Can you work these out from the model? Positions are in its coordinate system, mm. A direction names the side the tool comes from. Round coordinates to 2 decimals unless told otherwise and drop trailing zeros. Loops run counter-clockwise (first coordinate to the right, second up) from the corner with the lowest first, then second, coordinate; pieces in that order, holes last.
```python
from build123d import *

# Parameters (mm, degrees)
BASE_EXTRUDE_DEPTH = 10


with BuildPart() as part:
    # Sketch1 → Base-Extrude (new body)
    with BuildSketch(Plane.XY):
        with BuildLine():
            Line((89.567268983, -20.929801144), (19.452075124, 29.096679766))
            ThreePointArc((19.452075124, 29.096679766), (-16.495110953, 30.869261648), (-35, 0))
            ThreePointArc((-35, 0), (-43.227486122, -3.818813079), (-40.833333333, 4.930066486))
            Line((-40.833333333, 4.930066486), (-41.666666667, 9.860132972))
            ThreePointArc((-41.666666667, 9.860132972), (-46.454972244, -7.637626158), (-30, 0))
            ThreePointArc((-30, 0), (-14.170913912, 26.442110334), (16.612346594, 24.980591279))
            Line((16.612346594, 24.980591279), (86.66322331, -25))
            Line((86.66322331, -25), (89.567268983, -20.929801144))
        make_face()
    extrude(amount=BASE_EXTRUDE_DEPTH)


solid = part.part
```
(1) We'd pull the mould along Y, two halves only. Please class faces 1 (the flat face through (88.095, -22.993, 4.93)), 2 (the flat face through (25, 21, 10)), 3 (the cylindrical face through (-43, -4, 5)), 4 (the cylindrical face through (-16.026, 31.115, 4.93)): released by +Y, released by -Y, zero draft, split by the parting line, or undercut.
(2) Which directions (+Z, -Z, +X, -X, +Y, -Y) give clear straight access to the entire face, cutting with the end or side of a thin tool? Please do faces 5 (the flat face through (-41.244, 7.361, 4.93)), 6 (the cylindrical face through (-46.69, -7.43, 4.93)), 7 (the flat face through (51.15, 0.34, 4.93)).
(3) For pin 1 (12 mm diameter, centred on x = 21.5, y = 28.5, fed in from +Z); pin 2 (4 mm diameter, centred on x = 47, z = 5.5, fed in from -Y); pin 3 (4 mm diameter, centred on y = 5.5, z = 5.5, fed in from -X); pin 4 (3 mm diameter, centred on x = 59.5, z = 1.5, fed in from -Y), each with a flat end and sliding along its axis, tell me the tip position at first contact or that it passes through.
(4) If I drill on line 1 (Y direction, x = -40, z = 4.25); line 2 (X direction, y = 22, z = 6.75); line 3 (X direction, y = 16, z = 2.5), over which ranges is the centre line in solid material (lowest first)?
(5) Suppose I cut it at A-A (z = 5.5). Write out the boundary of the cut face in (x, y).
(6) Suppose I cut it at B-B (x = 78). Write out the boundary of the cut face in (y, z).
(7) Suppose I cut it at C-C (y = -19.5). Write out the boundary of the cut face in (x, z).
Check result:
1. face 1: released by -Y
1. face 2: zero draft
1. face 3: undercut
1. face 4: released by +Y
2. face 5: +Z, -Z, +Y
2. face 6: +Z, -Z
2. face 7: +Z, -Z, -Y
3. pin 1: stops at z = 10
3. pin 2: stops at y = 1.87
3. pin 3: stops at x = -49.37
3. pin 4: stops at y = -6.69
4. line 1: y = -10 to -5
4. line 2: x = -27.22 to -20.4, 20.79 to 29.4
4. line 3: x = -31.13 to -25.38, 29.2 to 37.81
5. outline: (-41.67, 9.86) arc R10 ccw (long way) to (-30, 0) arc R30 cw to (16.61, 24.98) - (86.66, -25) - (89.57, -20.93) - (19.45, 29.1) arc R35 ccw to (-35, 0) arc R5 cw (long way) to (-40.83, 4.93) - close
6. outline: (-18.82, 0) - (-12.68, 0) - (-12.68, 10) - (-18.82, 10) - close
7. outline: (78.95, 0) - (87.56, 0) - (87.56, 10) - (78.95, 10) - close
